Geometry: final body of the model. Coordinates: model frame, mm. A direction names the side the tool comes from. Coordinates: 2 decimals unless noted, no trailing zeros. Write each loop counter-clockwise with the first axis right and the second up, starting at its lowest first coordinate (ties: lowest second). Pieces come first, ordered by that corner, then holes. Notation, with made-up numbers: (89, -36) -> (109, -36) arc R16 cw to (109, -25) -> close; hole circle Ø8 at (7, 51). An arc over 180 degrees is marked (long way). One line per item, written item: value.
```python
from build123d import *

# Parameters (mm, degrees)
PORT_BORE_SKETCH_W = 16
PORT_BORE_SKETCH_H = 10.1125


with BuildPart() as part:
    # Bottle Sketch → Bottle (revolve)
    with BuildSketch(Plane.XY, mode=Mode.PRIVATE) as bottle_sk:
        Polygon((0, 0), (0, 16), (10, 16), (22, 26), (24.044450423, 39.329180823), (30.038475773, 51.75), (39.573593129, 62.415999231), (52, 70.600308295), (66.470857294, 75.745180054), (82, 77.5), (465.6, 77.5), (478.540952255, 74.859251537), (490.6, 67.116968793), (500.955339059, 54.800775542), (508.901270189, 38.75), (513.896291314, 20.058475995), (515.6, 0), align=None)
    revolve(bottle_sk.sketch.rotate(Axis((-1000, 0, 0), (1, 0, 0)), 90), axis=Axis((-1000, 0, 0), (1, 0, 0)))

    # Port Bore Sketch → Port Bore (revolve, cut)
    with BuildSketch(Plane.XY, mode=Mode.PRIVATE) as port_bore_sk:
        with Locations((7, 5.05625)):
            Rectangle(PORT_BORE_SKETCH_W, PORT_BORE_SKETCH_H)
    revolve(port_bore_sk.sketch.rotate(Axis((-1000, 0, 0), (1, 0, 0)), 90), axis=Axis((-1000, 0, 0), (1, 0, 0)), mode=Mode.SUBTRACT)


solid = part.part
```
(1) Pull-direction query (Z, two-part tool) for faces 3 (the cylindrical face through (7.6, 8.97, 4.67)), 4 (the conical face through (513.654, 12.758, -16.638)), 5 (the flat face through (0, -0.2, -10.4)), 6 (the flat face through (15, 0, 0)); classes: released by +Z, released by -Z, zero draft, split by the parting line, or undercut.
Responses:
face 3: undercut
face 4: split by the parting line
face 5: zero draft
face 6: undercut
(2) Line query: line 1 (Y direction, x = 8.75, z = 0); line 2 (Y direction, x = 415, z = -16); line 3 (Y direction, x = 10.25, z = 0). Output: solid intervals per line, ascending. Write a range as [from, to].
Responses:
line 1: y = [-16, -10.11], [10.11, 16]
line 2: y = [-75.83, 75.83]
line 3: y = [-16.21, -10.11], [10.11, 16.21]
(3) First-contact query: pin 1 (1.5 mm diameter, centred on x = 73, y = 37.5, fed in from -Z); pin 2 (1 mm diameter, centred on y = 54, z = -26, fed in from -X); pin 3 (1 mm diameter, centred on x = 90, z = -32, fed in from +Y). Flat tips, straight axial feed; report the tip coordinate or a pass-through.
Responses:
pin 1: stops at z = -67.09
pin 2: stops at x = 36.91
pin 3: stops at y = 70.81
(4) Reachability of faces 1 (the cylindrical face through (5.07, 15.62, -3.47)), 2 (the cylindrical face through (276.485, 68.756, 35.762)) from +Z, -Z, +X, -X, +Y, -Y: full face, straight path, thin tool, end or side. Return the list, or none.
Responses:
face 1: -X
face 2: +X, -X
(5) Section A-A (x = 224). Return the cut outline in (y, z).
Responses:
outline: circle Ø155 at (0, 0)
